Part model, mm, in its own coordinate system. Give positions to 0.01 mm unless a question says otherwise; leave off trailing zeros. Loops run counter-clockwise (first coordinate to the right, second up) from the corner with the lowest first, then second, coordinate; pieces in that order, holes last. Notation, with made-up numbers: (58, -39) -> (94, -39) arc R12 ccw to (94, -20) -> close; hole circle Ø11 at (10.5, 24). An arc over 180 degrees is marked (long way). Write item = value, one per line.
from build123d import *

# Parameters (mm, degrees)
SKETCH1_R           = 15
SKETCH1_R_2         = 16
BOSS_EXTRUDE1_DEPTH = 10


with BuildPart() as part:
    # Sketch1 → Boss-Extrude1 (new body)
    with BuildSketch(Plane.XY):
        with BuildLine():
            Line((88.973665961, 6.32455532), (68.973665961, 66.32455532))
            ThreePointArc((68.973665961, 66.32455532), (46.589060398, 79.706990918), (30.004417802, 59.579651831))
            ThreePointArc((30.004417802, 59.579651831), (23.077468599, 44.01959324), (6.67255707, 39.439535775))
            ThreePointArc((6.67255707, 39.439535775), (0, 40), (-6.67255707, 39.439535775))
            ThreePointArc((-6.67255707, 39.439535775), (-23.077468599, 44.01959324), (-30.004417802, 59.579651831))
            ThreePointArc((-30.004417802, 59.579651831), (-46.589060398, 79.706990918), (-68.973665961, 66.32455532))
            Line((-68.973665961, 66.32455532), (-88.973665961, 6.32455532))
            ThreePointArc((-88.973665961, 6.32455532), (-90, 0), (-88.973665961, -6.32455532))
            Line((-88.973665961, -6.32455532), (-68.973665961, -66.32455532))
            ThreePointArc((-68.973665961, -66.32455532), (-46.589060398, -79.706990918), (-30.004417802, -59.579651831))
            ThreePointArc((-30.004417802, -59.579651831), (-23.077468599, -44.01959324), (-6.67255707, -39.439535775))
            ThreePointArc((-6.67255707, -39.439535775), (0, -40), (6.67255707, -39.439535775))
            ThreePointArc((6.67255707, -39.439535775), (23.077468599, -44.01959324), (30.004417802, -59.579651831))
            ThreePointArc((30.004417802, -59.579651831), (46.589060398, -79.706990918), (68.973665961, -66.32455532))
            Line((68.973665961, -66.32455532), (88.973665961, -6.32455532))
            ThreePointArc((88.973665961, -6.32455532), (90, 0), (88.973665961, 6.32455532))
        make_face()
        with Locations((-50, -60)):
            Circle(SKETCH1_R, mode=Mode.SUBTRACT)
        with BuildLine():
            ThreePointArc((-16.5, -12.990381057), (-10.5, -18.186533479), (-3, -20.784609691))
            Line((-3, -20.784609691), (-3, -31.859064644))
            ThreePointArc((-3, -31.859064644), (-16, -27.712812921), (-26.090759323, -18.527608533))
            Line((-26.090759323, -18.527608533), (-16.5, -12.990381057))
        make_face(mode=Mode.SUBTRACT)
        with Locations((50, -60)):
            Circle(SKETCH1_R, mode=Mode.SUBTRACT)
        with BuildLine():
            Line((3, -31.859064644), (3, -20.784609691))
            ThreePointArc((3, -20.784609691), (10.5, -18.186533479), (16.5, -12.990381057))
            Line((16.5, -12.990381057), (26.090759323, -18.527608533))
            ThreePointArc((26.090759323, -18.527608533), (16, -27.712812921), (3, -31.859064644))
        make_face(mode=Mode.SUBTRACT)
        with BuildLine():
            ThreePointArc((-19.5, 7.794228634), (-21, 0), (-19.5, -7.794228634))
            Line((-19.5, -7.794228634), (-29.090759323, -13.331456111))
            ThreePointArc((-29.090759323, -13.331456111), (-32, 0), (-29.090759323, 13.331456111))
            Line((-29.090759323, 13.331456111), (-19.5, 7.794228634))
        make_face(mode=Mode.SUBTRACT)
        Circle(SKETCH1_R_2, mode=Mode.SUBTRACT)
        with BuildLine():
            ThreePointArc((-3, 20.784609691), (-10.5, 18.186533479), (-16.5, 12.990381057))
            Line((-16.5, 12.990381057), (-26.090759323, 18.527608533))
            ThreePointArc((-26.090759323, 18.527608533), (-16, 27.712812921), (-3, 31.859064644))
            Line((-3, 31.859064644), (-3, 20.784609691))
        make_face(mode=Mode.SUBTRACT)
        with Locations((-50, 60)):
            Circle(SKETCH1_R, mode=Mode.SUBTRACT)
        with BuildLine():
            ThreePointArc((19.5, -7.794228634), (21, 0), (19.5, 7.794228634))
            Line((19.5, 7.794228634), (29.090759323, 13.331456111))
            ThreePointArc((29.090759323, 13.331456111), (32, 0), (29.090759323, -13.331456111))
            Line((29.090759323, -13.331456111), (19.5, -7.794228634))
        make_face(mode=Mode.SUBTRACT)
        with BuildLine():
            ThreePointArc((16.5, 12.990381057), (10.5, 18.186533479), (3, 20.784609691))
            Line((3, 20.784609691), (3, 31.859064644))
            ThreePointArc((3, 31.859064644), (16, 27.712812921), (26.090759323, 18.527608533))
            Line((26.090759323, 18.527608533), (16.5, 12.990381057))
        make_face(mode=Mode.SUBTRACT)
        with Locations((70, 0)):
            Circle(SKETCH1_R, mode=Mode.SUBTRACT)
        with Locations((50, 60)):
            Circle(SKETCH1_R, mode=Mode.SUBTRACT)
        with Locations((-70, 0)):
            Circle(SKETCH1_R, mode=Mode.SUBTRACT)
    extrude(amount=BOSS_EXTRUDE1_DEPTH)


solid = part.part
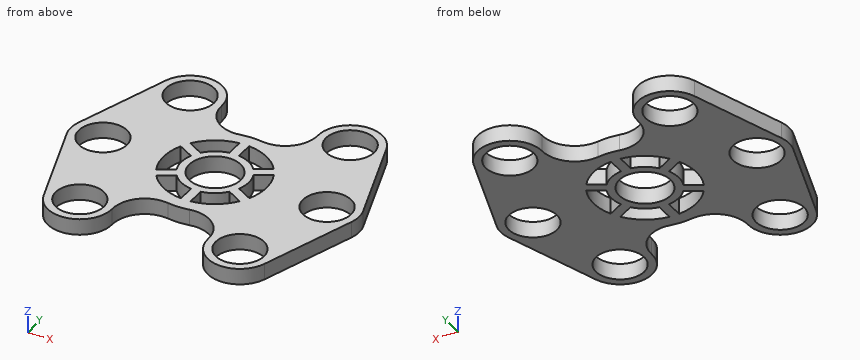
1) Slice it at B-B, the plane y = 49.5. List the corners of the cut face in (x, z), and give its area (3 significant figures).
Resolved:
outline = (-74.58, 0) -> (-60.71, 0) -> (-60.71, 10) -> (-74.58, 10) -> close; (-39.29, 0) -> (-27.52, 0) -> (-27.52, 10) -> (-39.29, 10) -> close; (27.52, 0) -> (39.29, 0) -> (39.29, 10) -> (27.52, 10) -> close; (60.71, 0) -> (74.58, 0) -> (74.58, 10) -> (60.71, 10) -> close
area = 513 mm²
2) Slice it at C-C, the plane x = 71. List the corners of the cut face in (y, z).
Resolved:
outline = (-60.25, 0) -> (-14.97, 0) -> (-14.97, 10) -> (-60.25, 10) -> close; (14.97, 0) -> (60.25, 0) -> (60.25, 10) -> (14.97, 10) -> close
3) Slice it at A-A, the plane x = -50. List the corners of the cut face in (y, z).
Resolved:
outline = (-80, 0) -> (-75, 0) -> (-75, 10) -> (-80, 10) -> close; (-45, 0) -> (45, 0) -> (45, 10) -> (-45, 10) -> close; (75, 0) -> (80, 0) -> (80, 10) -> (75, 10) -> close
4) Slice it at D-D, the plane y = -2. List the corners of the cut face in (x, z), and give its area (3 significant figures).
Resolved:
outline = (-89.9, 0) -> (-84.87, 0) -> (-84.87, 10) -> (-89.9, 10) -> close; (-55.13, 0) -> (-31.94, 0) -> (-31.94, 10) -> (-55.13, 10) -> close; (-20.9, 0) -> (-15.87, 0) -> (-15.87, 10) -> (-20.9, 10) -> close; (15.87, 0) -> (20.9, 0) -> (20.9, 10) -> (15.87, 10) -> close; (31.94, 0) -> (55.13, 0) -> (55.13, 10) -> (31.94, 10) -> close; (84.87, 0) -> (89.9, 0) -> (89.9, 10) -> (84.87, 10) -> close
area = 665 mm²
5) Drop flat-ended pins along their axis: P1, Ø5, axis at y = -24, z = 3, coming from the +X side; P2, Ø5, axis at y = 62.5, z = 8, coming from the -X side; P3, Ø5, axis at x = 70.5, z = 1, coming from the +Y side. Give the stop position or say it passes through.
Resolved:
P1 = 83.92
P2 = -71.08
P3 = 68.72
6) Drill centre lines: line 1 along Y through (x, z) = (-50, 4); line 2 along X through (y, z) = (60.5, 7); line 3 along X through (y, z) = (-69, 6). Where is each one in solid material? Low to high. Write a range as [from, to].
Resolved:
line_1 = [-80, -75], [-45, 45], [75, 80]
line_2 = [-70.92, -64.99], [-35.01, -30.01], [30.01, 35.01], [64.99, 70.92]
line_3 = [-67.86, -62], [-38, -32.14], [32.14, 38], [62, 67.86]
